from build123d import *

# Parameters (mm, degrees)
CROQUIS1_W              = 350
CROQUIS1_H              = 20
SALIENTE_EXTRUIR1_DEPTH = 45
CROQUIS2_R              = 11.125
CORTAR_EXTRUIR1_DEPTH   = 182.796589627
CROQUIS3_R              = 11.125
CORTAR_EXTRUIR3_DEPTH   = 182.796589627


with BuildPart() as part:
    # Croquis1 → Saliente-Extruir1 (new body)
    with BuildSketch(Plane(origin=(0, 0, 0), x_dir=(1, 0, 0), z_dir=(0, 1, 0))):
        Rectangle(CROQUIS1_W, CROQUIS1_H)
    extrude(amount=SALIENTE_EXTRUIR1_DEPTH)

    # Croquis2 → Cortar-Extruir1 (cut, through all)
    with BuildSketch(Plane(origin=(0, 0, -10), x_dir=(-1, 0, 0), z_dir=(0, 0, -1))):
        with Locations((-143.9, 21.1)):
            Circle(CROQUIS2_R)
    cortar_extruir1 = extrude(amount=-CORTAR_EXTRUIR1_DEPTH, mode=Mode.SUBTRACT)

    # Simetría1: Cortar-Extruir1 across plane
    add(cortar_extruir1.mirror(Plane(origin=(0, 0, 0), x_dir=(0, 0, 1), z_dir=(1, 0, 0))), mode=Mode.SUBTRACT)

    # Croquis3 → Cortar-Extruir3 (cut, through all)
    with BuildSketch(Plane.XY.offset(10)):
        Polygon((-175, 0), (0, 0), (25, 0), (25, 15), (-25, 15), (-25, 30), (25, 30), (25, 45), (-175, 45), align=None)
        with Locations((-143.9, 21.1)):
            Circle(CROQUIS3_R, mode=Mode.SUBTRACT)
    extrude(amount=-CORTAR_EXTRUIR3_DEPTH, mode=Mode.SUBTRACT)


solid = part.part
Model file for the job. Use its own axes, mm. A direction names the side the tool comes from. Round coordinates to 2 decimals unless told otherwise and drop trailing zeros. Loops run counter-clockwise (first coordinate to the right, second up) from the corner with the lowest first, then second, coordinate; pieces in that order, holes last. Notation, with made-up numbers: (73.25, 86.5) -> (85.25, 86.5) arc R10 cw to (85.25, 90.5) -> close; hole circle Ø9 at (-15.5, 57.5). An arc over 180 degrees is marked (long way). Answer as CSV lines item,"result". Start each with the question number.
1) Pin check, flat tips, straight feed: P1, Ø4.5, axis at y = 37.5, z = 3, coming from the -X side; P2, Ø10, axis at x = -1.5, z = 3, coming from the +Y side; P3, Ø10, axis at x = 4.5, z = -1, coming from the -Y side. Stop position of each tip, or through.
2) Slice it at D-D (y = 5.5). List the corners of the cut face in (x, z).
3) Probe line 1 along Y through (x, z) = (143.9, 5.5) (3 decimals); line 2 along X through (y, z) = (42, -0.5); line 3 along X through (y, z) = (14.5, -0.5). List the from-to ranges inside material, lowest first.
4) Slice it at A-A (y = 21.1). List the corners of the cut face in (x, z) (3 decimals), plus the area to 4 significant figures.
5) Slice it at B-B (x = 143.9). List the corners of the cut face in (y, z) (3 decimals), plus the area to 3 significant figures.
6) Mould opens along Y. For faces 1 (the face through (0, 30, 0)), 2 (the face through (133.29, 24.44, -0.14)), 3 (the face through (-25, 22, 0)), 4 (the face through (99, 0, 0)) say: +Y half, -Y half, draft (parallel to the pull), parting line (faces both ways), or undercut.
7) Tool access for faces 5 (the face through (74, 22, -10)), 6 (the face through (25, 37, 0)), 7 (the face through (25, 7, 0)): list every direction of +Z, -Z, +X, -X, +Y, -Y with a clear straight run to the whole face (end or side of a thin tool).
8) Slice it at C-C (z = 2). List the corners of the cut face in (x, y) (3 decimals).
Filled in:
1,P1,"stops at x = 25"
1,P2,"stops at y = 30"
1,P3,"stops at y = 15"
2,outline,"(25, -10) -> (175, -10) -> (175, 10) -> (25, 10) -> close"
3,line 1,"y = 0 to 9.975, 32.225 to 45"
3,line 2,"x = 25 to 175"
3,line 3,"x = 25 to 134.94, 152.86 to 175"
4,outline,"(-25, -10) -> (132.775, -10) -> (132.775, 10) -> (-25, 10) -> close; (155.025, -10) -> (175, -10) -> (175, 10) -> (155.025, 10) -> close"
4,area,"3,555 mm2"
5,outline,"(0, -10) -> (9.975, -10) -> (9.975, 10) -> (0, 10) -> close; (32.225, -10) -> (45, -10) -> (45, 10) -> (32.225, 10) -> close"
5,area,"455 mm2"
6,face 1,"+Y half"
6,face 2,"undercut"
6,face 3,"draft"
6,face 4,"-Y half"
7,face 5,"-Z, +X, -X, +Y, -Y"
7,face 6,"+Z, -Z, -X, +Y"
7,face 7,"+Z, -Z, -X, -Y"
8,outline,"(-25, 15) -> (25, 15) -> (25, 0) -> (175, 0) -> (175, 45) -> (25, 45) -> (25, 30) -> (-25, 30) -> close; hole circle Ø22.25 at (143.9, 21.1)"
